For this review, take the finished solid that the model builds, in its own axes (mm). Face numbers are marked on the shaded views. A direction names the side the tool comes from. Round coordinates to 2 decimals unless told otherwise and drop trailing zeros. Order: outer loops, then holes, each group sorted by start corner. A loop starts at its lowest first (then second) coordinate and runs counter-clockwise, first axis right, second up.
Autodesk Inventor part; units mm, degrees
ref_plane "YZ Plane" through (0, 0, 0) normal (1, 0, 0) x (0, 1, 0)
ref_plane "XZ Plane" through (0, 0, 0) normal (0, 1, 0) x (-1, 0, 0)
ref_plane "XY Plane" through (0, 0, 0) normal (0, 0, 1) x (1, 0, 0)
sketch "Sketch1" plane through (0, 0, 0) normal (0, 0, 1) x (1, 0, 0)
  line L0 (0, 0) -> (3, 0)
  line L1 (3, 0) -> (3, 25)
  line L2 (3, 25) -> (0, 25)
  line L3 (0, 25) -> (0, 0)
  line L4 (34, 25) -> (38, 25)
  line L5 (38, 25) -> (38, 0)
  line L6 (38, 0) -> (34, 0)
  line L7 (34, 0) -> (34, 25)
  line L8 (0, 25) -> (38, 25)
  line L9 (38, 25) -> (38, 45)
  line L10 (38, 45) -> (0, 45)
  line L11 (0, 45) -> (0, 25)
  line L12 (0, 25) -> (0, 30)
  line L13 (0, 30) -> (28, 45)
  line L14 (28, 45) -> (38, 45)
  point P0 (34, 25)
  dimension "d0" = 3
  dimension "d1" = 25
  dimension "d2" = 4
  dimension "d3" = 25
  dimension "d4" = 31
  dimension "d5" = 38
  dimension "d6" = 20
  dimension "d7" = 5
  dimension "d10" = 10
extrude "Extrusion1" add sketch "Sketch1" along normal blind 17 contours L3 L2 L1 L0 | L11 L13 L10 L9 L4 L8 L2 | L4 L5 L6 L7
sketch "Sketch2" plane through (38, 0, 0) normal (1, 0, 0) x (0, 0, -1)
  line L0 (0, 25) -> (-17, 25)
  line L1 (0, 0) -> (0, 45)
  line L2 (-17, 25) -> (0, 25)
  line L3 (0, 25) -> (0, 45)
  line L4 (0, 45) -> (-17, 45)
  line L5 (-17, 45) -> (-17, 25)
  circle A0 centre (-8.5, 30) radius 1.5
  circle A1 centre (-8.5, 40) radius 1.5
  dimension "d11" = 3
  dimension "d12" = 3
  dimension "d13" = 5
  dimension "d15" = 8.5
  dimension "d16" = 5
  dimension "d19" = 17
  dimension "d20" = 8.5
  dimension "d21" = 20
extrude "Extrusion2" cut sketch "Sketch2" against normal blind 10 contours A0 | A1
sketch "Sketch3" plane through (38, 0, 0) normal (1, 0, 0) x (0, 0, -1)
  circle A0 centre (-8.5, 5) radius 3.75
  line L0 (0, 0) -> (-17, 0)
  line L1 (0, 0) -> (0, 45)
  point P0 (-8.5, 0)
  dimension "d22" = 7.5
  dimension "d23" = 5
  dimension "d24" = 8.5
extrude "Extrusion3" cut sketch "Sketch3" against normal up to surface (4 mm away)
fillet "Fillet1" radius 8.5 4 edges at (36, 0, 17) (1.5, 0, 17) (1.5, 0, 0) (36, 0, 0)
sketch "Sketch4" plane through (0, 30, 0) normal (-1, 0, 0) x (0, 0, 1)
  circle A0 centre (8.5, -25) radius 2.5
  arc A1 (0, -21.5) -> (17, -21.5) centre (8.5, -21.5) ccw
  line L0 (17, 0) -> (17, -21.5)
  point P0 (0, -30)
  point P1 (8.5, -30)
  dimension "d28" = 5
  dimension "d29" = 5
  dimension "d30" = 8.5
extrude "Extrusion4" cut sketch "Sketch4" against normal up to surface (3 mm away)
sketch "Sketch5" plane through (38, 45, 17) normal (1, 0, 0) x (0, 0, -1)
  circle A0 centre (8.5, -40) radius 3.75
  circle A1 centre (8.5, -40) radius 3.5
  circle A2 centre (8.5, -25) radius 2
  circle A3 centre (8.5, -40) radius 3.75
  line L0 (10.4863, -24.7667) -> (12.2244, -39.5625)
  line L1 (6.5137, -24.7667) -> (4.7756, -39.5625)
  point P0 (17, -45)
  dimension "d33" = 4
  dimension "d34" = 15
  dimension "d35" = 0
extrude "Extrusion5" cut sketch "Sketch5" against normal blind 2 contours A0 | A0 L1 A2 L0 | A2 | A1
properties part number "juncao6"
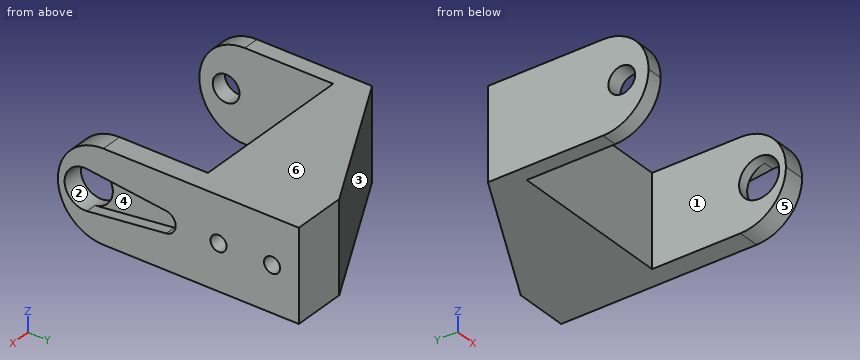
Q1. Tool access review of the marked faces 1, 2 and 3: name each direction out of +Z, -Z, +X, -X, +Y, -Y from which nothing blocks a thin tool from reaching the whole face with its end or side.
Q2. Wall thickness on line 1 (Y direction, x = 37.1, z = 8.5); line 2 (X direction, y = 9, z = 3.5); line 3 (Y direction, x = 32, z = 7.25): over which ranges is each line inside the solid? List them lowest first.
Q3. Take a section at A-A, the plane z = 9. State the section outline as (x, y) points.
Q4. Take a section at C-C, the plane y = 40. State the section outline as (x, z) points, plus the area to 3 significant figures.
Q5. Take a section at D-D, the plane z = 15.75. State the section outline as (x, y) points.
Q6. Clearance check with flat-ended pins moving along their axes: pin 1 (4.5 mm diameter, centred on y = 5, z = 8.5, fed in from -X); pin 2 (10 mm diameter, centred on x = 10.5, z = 8.5, fed in from -Y); pin 3 (0.9 mm diameter, centred on y = 30, z = 8, fed in from +X); pin 4 (2 mm diameter, centred on y = 18, z = 9.5, fed in from +X). State where each tip first meets the part, or that it passes through.
Q7. Mouldability with a two-part tool opening along Y and no side actions: class the marked faces 4, 5 and 6 as +Y half, -Y half, draft (parallel to the pull), parting line (faces both ways), or undercut.
Q8. Take a section at B-B, the plane y = 6.5. State the section outline as (x, z) points, plus the area to 3 significant figures.
Working result:
1. face 1: +Z, -Z, -Y
1. face 2: +X
1. face 3: +Z, -Z, -X, +Y
2. line 1: y = 0 to 1.25, 22 to 28.5, 31.5 to 38.5, 41.5 to 45
2. line 2: x = 0 to 3, 34 to 38
2. line 3: y = 25 to 29.17, 30.83 to 39.17, 40.83 to 45
3. outline: (0, 0.01) - (3, 0.01) - (3, 2.55) - (0, 2.55) - close; (0, 7.45) - (3, 7.45) - (3, 25) - (34, 25) - (34, 8.72) - (36, 8.72) - (36, 21.94) - (38, 21.94) - (38, 28.59) - (28, 28.59) - (28, 31.41) - (38, 31.41) - (38, 38.59) - (28, 38.59) - (28, 41.41) - (38, 41.41) - (38, 45) - (28, 45) - (0, 30) - close; (34, 0.01) - (38, 0.01) - (38, 1.28) - (34, 1.28) - close
4. outline: (18.67, 0) - (38, 0) - (38, 7) - (28, 7) - (28, 10) - (38, 10) - (38, 17) - (18.67, 17) - close
4. area: 299 mm2
5. outline: (0, 4.06) - (3, 4.06) - (3, 25) - (34, 25) - (34, 4.06) - (38, 4.06) - (38, 45) - (28, 45) - (0, 30) - close
6. pin 1: passes through
6. pin 2: stops at y = 25
6. pin 3: stops at x = 28
6. pin 4: stops at x = 36
7. face 4: undercut
7. face 5: -Y half
7. face 6: draft
8. outline: (0, 0.24) - (3, 0.24) - (3, 6.5) - (0, 6.5) - close; (0, 10.5) - (3, 10.5) - (3, 16.76) - (0, 16.76) - close; (34, 0.24) - (38, 0.24) - (38, 4.9) - (36, 4.9) - (36, 5.06) - (34, 5.06) - close; (34, 11.94) - (36, 11.94) - (36, 12.1) - (38, 12.1) - (38, 16.76) - (34, 16.76) - close
8. area: 75.5 mm2
